The drawing under review shows one solid part. Ordinate dimensions are in mm from its lowest x, y, z. Coordinates: 2 decimals unless noted, no trailing zeros. Order: outer loops, then holes, each group sorted by start corner. A loop starts at its lowest first (then second) coordinate and runs counter-clockwise, first axis right, second up.
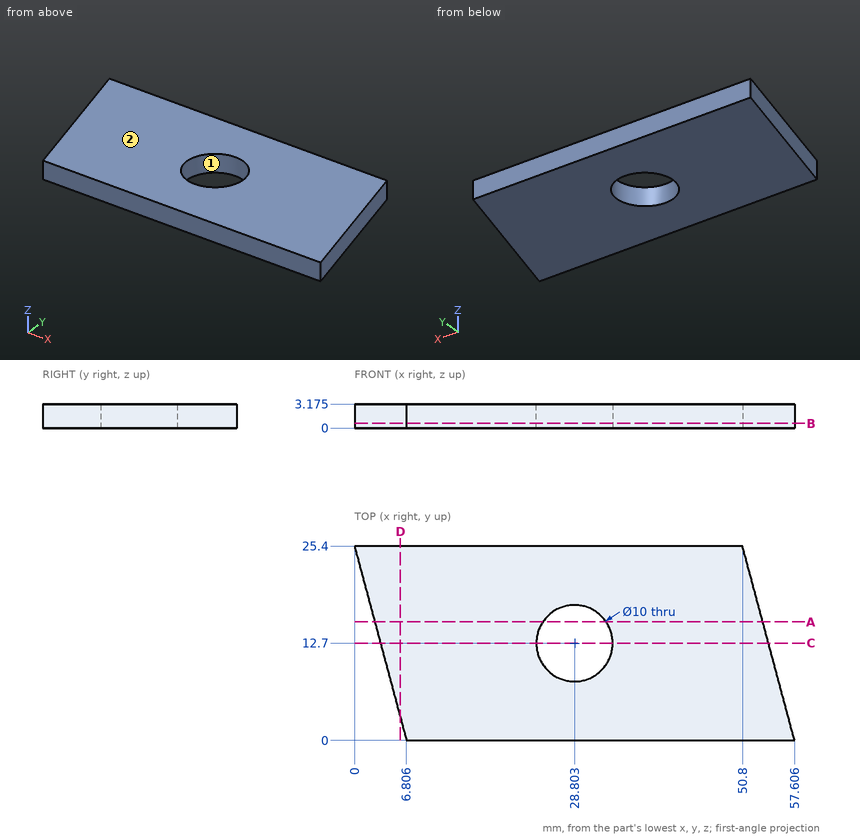
(1) Wall thickness on probe 1 along X at (y, z) = (19.5, 0.1); probe 2 along X at (y, z) = (15.75, 2) (1 decimal); probe 3 along X at (y, z) = (6, 3): over which ranges is each line inside the solid? List them lowest first.
A:
probe 1: x = 1.58 to 52.38
probe 2: x = 2.6 to 24.8, 32.8 to 53.4
probe 3: x = 5.2 to 56
(2) Draft analysis for pull direction X (two halves, no side actions). For the marked faces 1 and 2, state which applies: released by +X, released by -X, zero draft, split by the parting line, or undercut.
A:
face 1: undercut
face 2: zero draft
(3) We need section B-B, the plane z = 0.65. Write out the cut boundary in (x, y).
A:
outline: (0, 25.4) - (6.81, 0) - (57.61, 0) - (50.8, 25.4) - close; hole circle Ø10 at (28.8, 12.7)
(4) We need section A-A, the plane y = 15.5. Write out the cut boundary in (x, z) (1 decimal).
A:
outline: (2.7, 0) - (24.7, 0) - (24.7, 3.2) - (2.7, 3.2) - close; (32.9, 0) - (53.5, 0) - (53.5, 3.2) - (32.9, 3.2) - close
(5) We need section D-D, the plane x = 6. Write out the cut boundary in (y, z) (3 decimals), and give its area (3 significant figures).
A:
outline: (3.008, 0) - (25.4, 0) - (25.4, 3.175) - (3.008, 3.175) - close
area: 71.1 mm2
(6) We need section C-C, the plane y = 12.7. Write out the cut boundary in (x, z) (3 decimals), and give its area (3 significant figures).
A:
outline: (3.403, 0) - (23.803, 0) - (23.803, 3.175) - (3.403, 3.175) - close; (33.803, 0) - (54.203, 0) - (54.203, 3.175) - (33.803, 3.175) - close
area: 130 mm2
